from build123d import *

# Parameters (mm, degrees)
ESQUISSE1_W          = 360
ESQUISSE1_H          = 220
BOSS_EXTRU_1_DEPTH   = 3
M6_CLEARANCE_HOLE1_D = 6.6
CHAMFER1_SIZE        = 5


with BuildPart() as part:
    # Esquisse1 → Boss.-Extru.1 (new body)
    with BuildSketch(Plane(origin=(0, 0, 0), x_dir=(1, 0, 0), z_dir=(0, 1, 0))):
        Rectangle(ESQUISSE1_W, ESQUISSE1_H)
    extrude(amount=BOSS_EXTRU_1_DEPTH)

    # M6 Clearance Hole1 (through all)
    with Locations(Plane(origin=(0, 0, 0), x_dir=(-1, 0, 0), z_dir=(0, -1, 0))):
        with Locations((-170, 100), (0, 100), (170, 100), (0, 0), (170, 0), (0, -100), (170, -100), (-170, 0), (-170, -100)):
            Hole(M6_CLEARANCE_HOLE1_D / 2)

    # Chamfer1
    chamfer1_edges = [part.edges().sort_by_distance(p)[0] for p in [
        (180, 1.5, 110),
        (-180, 1.5, 110),
        (-180, 1.5, -110),
        (180, 1.5, -110),
    ]]
    chamfer(chamfer1_edges, length=CHAMFER1_SIZE)


solid = part.part
CAD build for the part. Positions are in the model's coordinates, mm. Coordinates: 2 decimals unless noted, no trailing zeros. Return JSON: item names as keys, results as strings.
Item 1: Probe line 1 (X direction, y = 2.1, z = -100); line 2 (Z direction, x = -170, y = 1); line 3 (Z direction, x = 1, y = 1.9). List the from-to ranges inside material, lowest first. Write a range as from..to.
Findings below:
{"line 1": "x = -180..-173.3, -166.7..-3.3, 3.3..166.7, 173.3..180", "line 2": "z = -110..-103.3, -96.7..-3.3, 3.3..96.7, 103.3..110", "line 3": "z = -110..-103.14, -96.86..-3.14, 3.14..96.86, 103.14..110"}
Item 2: Two-plate mould, pull along X, no slides. Class faces 1 (the cylindrical face through (1.774, 1.521, -102.783)), 2 (the flat face through (-3, 3, 23)): +X half, -X half, draft (parallel to the pull), parting line (faces both ways), or undercut.
Findings below:
{"face 1": "undercut", "face 2": "draft"}
Item 3: Drop a flat-ended pin along its axis: pin 1 Ø6 at (x, z) = (-170, 0) entering from +Y. Give the stop position or say it passes through.
Findings below:
{"pin 1": "passes through"}
